from build123d import *

# Parameters (mm, degrees)
BOSS_EXTRU_1_DEPTH      = 3
ESQUISSE2_R             = 3
ENL_V_MAT_EXTRU_1_DEPTH = 10
ESQUISSE7_R             = 4
ENL_V_MAT_EXTRU_2_DEPTH = 10
ESQUISSE8_W             = 10.5
ESQUISSE8_H             = 10.5
ENL_V_MAT_EXTRU_3_DEPTH = 10


with BuildPart() as part:
    # Esquisse1 → Boss.-Extru.1 (new body)
    with BuildSketch(Plane.XY):
        with BuildLine():
            Line((118.101682981, 78.402253408), (267.271682981, 78.402253408))
            ThreePointArc((267.271682981, 78.402253408), (277.878284699, 82.795651691), (282.271682981, 93.402253408))
            Line((282.271682981, 93.402253408), (282.271682981, 137.632253408))
            ThreePointArc((282.271682981, 137.632253408), (280.807216887, 141.167787314), (277.271682981, 142.632253408))
            Line((277.271682981, 142.632253408), (108.101682981, 142.632253408))
            ThreePointArc((108.101682981, 142.632253408), (104.566149075, 141.167787314), (103.101682981, 137.632253408))
            Line((103.101682981, 137.632253408), (103.101682981, 93.402253408))
            ThreePointArc((103.101682981, 93.402253408), (107.495081263, 82.795651691), (118.101682981, 78.402253408))
        make_face()
    extrude(amount=BOSS_EXTRU_1_DEPTH)

    # Esquisse2 → Enlèv. mat.-Extru.1 (cut)
    with BuildSketch(Plane(origin=(0, 0, 0), x_dir=(-1, 0, 0), z_dir=(0, 0, -1))):
        with Locations((-111.741682981, 113.692253408)):
            Circle(ESQUISSE2_R)
        with Locations((-111.721682981, 86.402253408)):
            Circle(ESQUISSE2_R)
        with Locations((-248.301682981, 123.122253408)):
            Circle(ESQUISSE2_R)
        with Locations((-274.271682981, 85.752253408)):
            Circle(ESQUISSE2_R)
    extrude(amount=-ENL_V_MAT_EXTRU_1_DEPTH, mode=Mode.SUBTRACT)

    # Esquisse7 → Enlèv. mat.-Extru.2 (cut)
    with BuildSketch(Plane.XY.offset(3)):
        with Locations((100.601682981, 103.122253408)):
            Circle(ESQUISSE7_R)
        with Locations((284.771682981, 104.902253408)):
            Circle(ESQUISSE7_R)
        with Locations((284.771682981, 132.442253408)):
            Circle(ESQUISSE7_R)
    extrude(amount=-ENL_V_MAT_EXTRU_2_DEPTH, mode=Mode.SUBTRACT)

    # Esquisse8 → Enlèv. mat.-Extru.3 (cut)
    with BuildSketch(Plane(origin=(0, 0, 0), x_dir=(-1, 0, 0), z_dir=(0, 0, -1))):
        with Locations((-232.021682981, 90.852253408)):
            Rectangle(ESQUISSE8_W, ESQUISSE8_H)
    extrude(amount=-ENL_V_MAT_EXTRU_3_DEPTH, mode=Mode.SUBTRACT)


solid = part.part
Work out the finished part from the listing and answer in its coordinate system (mm). A direction names the side the tool comes from. Coordinates: 2 decimals unless noted, no trailing zeros. Order: outer loops, then holes, each group sorted by start corner. A loop starts at its lowest first (then second) coordinate and runs counter-clockwise, first axis right, second up. Notation, with made-up numbers: (14.25, 52.5) - (53.25, 52.5) arc R17 ccw to (53.25, 63.5) - close; hole circle Ø5 at (35.25, 52). An arc over 180 degrees is marked (long way). Put each result on its own line as item: value. Start each with the question number.
1) Find the intervals of material crossed by line 1 (X direction, y = 86, z = 0.4); line 2 (X direction, y = 84.5, z = 2.2); line 3 (X direction, y = 94, z = 2.45), in increasing order. Write a range as from..to.
2) For a pull along Y with two mould halves and no side action, classify faces 1 (the flat face through (192, 78.402, 1)), 2 (the cylindrical face through (104.6, 141.2, 1.5)), 3 (the flat face through (191, 111, 3)), 4 (the cylindrical face through (251.3, 123.25, 1.48)) as released by +Y, released by -Y, zero draft, split by the parting line, or undercut.
3) For faces 5 (the flat face through (194, 142.632, 1)), 6 (the flat face through (237.272, 91, 1)), determine the directions among +Z, -Z, +X, -X, +Y, -Y from which every point of the face is accessible in a straight line to the end or side of a thin tool.
4) Flat-ended cylindrical pins translate along their axes: pin 1 (1.5 mm diameter, centred on y = 89, z = 1, fed in from -X); pin 2 (5 mm diameter, centred on x = 167, y = 89, fed in from -Z); pin 3 (3.5 mm diameter, centred on x = 111.74, y = 113.69, fed in from -Z). Find the tip coordinate at first contact, or state that the pin passes through.
5) Find section A-A (z = 1). Give the vertices of the cut face in (x, y).
Results list:
1. line 1: x = 105.06..108.75, 114.69..226.77, 237.27..271.28, 277.26..280.32
1. line 2: x = 106.03..109.4, 114.04..271.55, 277..279.34
1. line 3: x = 103.1..226.77, 237.27..282.27
2. face 1: released by -Y
2. face 2: released by +Y
2. face 3: zero draft
2. face 4: undercut
3. face 5: +Z, -Z, +X, -X, +Y
3. face 6: +Z, -Z
4. pin 1: stops at x = 103.55
4. pin 2: stops at z = 0
4. pin 3: passes through
5. outline: (103.1, 93.4) arc R15 ccw to (118.1, 78.4) - (267.27, 78.4) arc R15 ccw to (282.27, 93.4) - (282.27, 101.78) arc R4 cw to (282.27, 108.02) - (282.27, 129.32) arc R4 cw to (282.27, 135.56) - (282.27, 137.63) arc R5 ccw to (277.27, 142.63) - (108.1, 142.63) arc R5 ccw to (103.1, 137.63) - (103.1, 106.24) arc R4 cw to (103.1, 100) - close; hole circle Ø6 at (111.72, 86.4); hole circle Ø6 at (111.74, 113.69); hole (226.77, 85.6) - (237.27, 85.6) - (237.27, 96.1) - (226.77, 96.1) - close; hole circle Ø6 at (248.3, 123.12); hole circle Ø6 at (274.27, 85.75)
